Check sheet for the drawn part. Datum: minimum x, y, z corner. Units: mm. Round coordinates to 2 decimals unless told otherwise and drop trailing zeros. Write each loop counter-clockwise with the first axis right and the second up, starting at its lowest first coordinate (ties: lowest second). Pieces come first, ordered by that corner, then holes. Notation, with made-up numbers: (-3, -20) - (42, -20) arc R17 cw to (42, -14) - close; hole circle Ø7 at (-24, -12). An arc over 180 degrees is marked (long way). Answer as a JSON object with one key per item and string values. Group by question number.
Item 1: Thickness scan on line 1 (Z direction, x = 75, y = 15.25); line 2 (X direction, y = 15.75, z = 90); line 3 (X direction, y = 22.5, z = 78). Record the ranges inside material, lowest first.
Item 2: Sectioned sample at D-D on x = 195.5. Record the boundary of the cut face in (y, z).
Item 3: Gauge pin test, flat ends, axial feed: P1, Ø8, axis at y = 8.5, z = 139, coming from the -X side; P2, Ø4, axis at x = 183.5, y = 16, coming from the +Z side; P3, Ø5, axis at x = 171.5, y = 3.5, coming from the -Z side. Record the tip position at first contact, or that the pin passes through.
Item 4: Sectioned sample at A-A on z = 75. Record the boundary of the cut face in (x, y), plus the area to 3 significant figures.
Item 5: Sectioned sample at C-C on y = 16.75. Record the boundary of the cut face in (x, z), plus the area to 3 significant figures.
Item 6: Release check for a two-part mould opening along X. For the marked faces 1, 2 and 3 record: pulls with the +X half, pulls with the -X half, needs draft (parallel to the pull), parting line crosses it, or undercut.
Item 7: Sectioned sample at B-B on x = 75. Record the boundary of the cut face in (y, z).
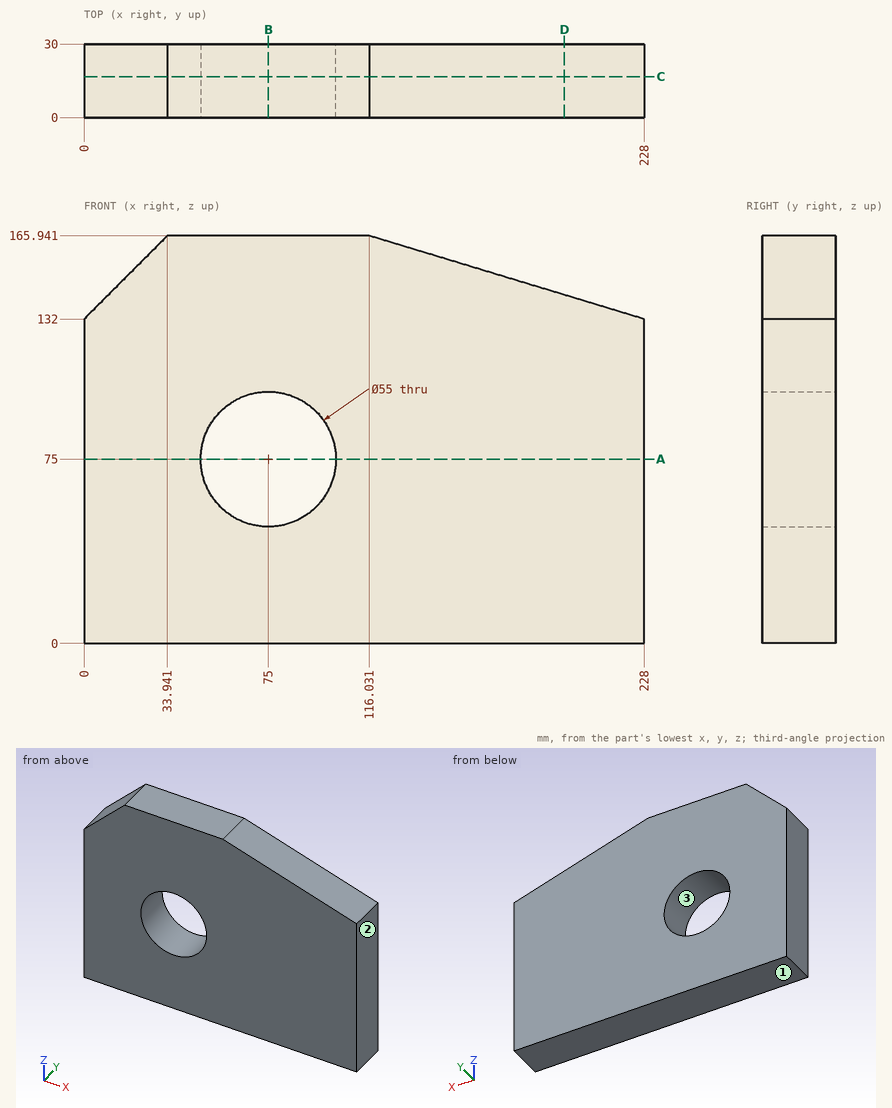
Completed:
{
 "1": {"line 1": "0 to 47.5, 102.5 to 165.94", "line 2": "0 to 51.95, 98.05 to 228", "line 3": "0 to 47.66, 102.34 to 228"},
 "2": {"outline": "(0, 0) - (30, 0) - (30, 141.85) - (0, 141.85) - close"},
 "3": {"P1": "x = 3", "P2": "z = 146.1", "P3": "z = 0"},
 "4": {"outline": "(0, 0) - (47.5, 0) - (47.5, 30) - (0, 30) - close; (102.5, 0) - (228, 0) - (228, 30) - (102.5, 30) - close", "area": "5,190 mm²"},
 "5": {"outline": "(0, 0) - (228, 0) - (228, 132) - (116.03, 165.94) - (33.94, 165.94) - (0, 132) - close; hole circle Ø55 at (75, 75)", "area": "33,000 mm²"},
 "6": {"face 1": "needs draft", "face 2": "pulls with the +X half", "face 3": "undercut"},
 "7": {"outline": "(0, 0) - (30, 0) - (30, 47.5) - (0, 47.5) - close; (0, 102.5) - (30, 102.5) - (30, 165.94) - (0, 165.94) - close"}
}
